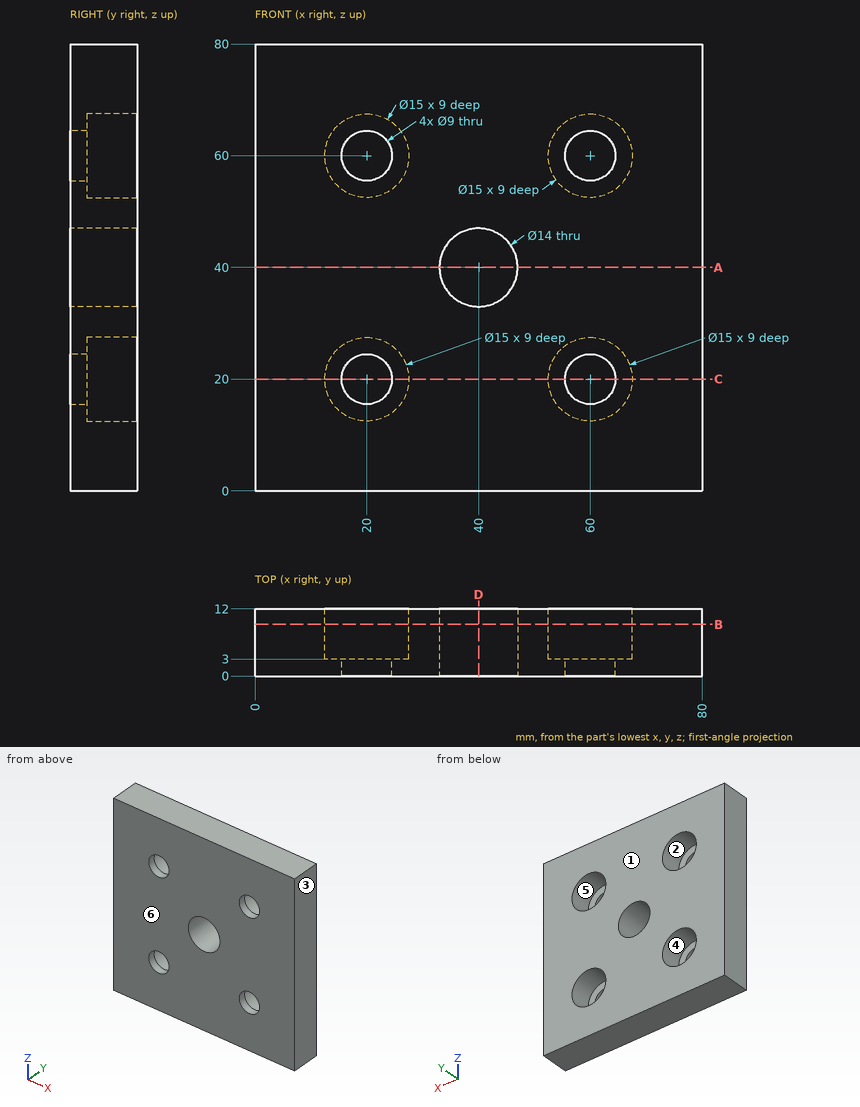
Geometry check sheet. Reference: drawing and pictorial views, mm from the part's lowest x, y, z. A direction names the side the tool comes from. Give positions to 0.01 mm unless a question says otherwise; leave off trailing zeros. Write each loop counter-clockwise with the first axis right and the second up, starting at its lowest first coordinate (ties: lowest second). Pieces come first, ordered by that corner, then holes. Notation, with made-up numbers: M -16,0.5 L -10,0.5 A26 cw -10,16.5 Z; hole C 4,-30 d2. An arc over 180 degrees is marked long. Put each result on its own line as item: value. Start each with the question number.
1. Scan lines: line 1 along X through (y, z) = (2.05, 20); line 2 along X through (y, z) = (7.75, 20); line 3 along Z through (x, y) = (39.5, 7.75). Record each from-to range of solid material in increasing order. Write a range as [from, to].
2. Section check A-A (z = 40). Record the cut outline in (x, y).
3. Go/stop test with flat-tipped pins: pin 1 Ø12.5 at (x, z) = (40, 40) entering from +Y; pin 2 Ø12 at (x, z) = (17.5, 16.5) entering from +Y; pin 3 Ø4.5 at (x, z) = (16.5, 63) entering from +Y. Record where each tip stops, or that it passes through.
4. Section check C-C (z = 20). Record the cut outline in (x, y), and give its area (3 significant figures).
5. Set-up check for the marked faces 1 and 2: record each of +Z, -Z, +X, -X, +Y, -Y from which the full face is reachable in a straight line by a thin tool's end or side.
6. Draft check along X on the marked faces 3, 4, 5 and 6. Enter one of: +X half, -X half, draft (parallel to the pull), parting line (faces both ways), or undercut.
7. Section check D-D (x = 40). Record the cut outline in (y, z), and give its area (3 significant figures).
8. Section check B-B (y = 9.25). Record the cut outline in (x, z), and give its area (3 significant figures).
Answer list:
1. line 1: [0, 15.5], [24.5, 55.5], [64.5, 80]
1. line 2: [0, 12.5], [27.5, 52.5], [67.5, 80]
1. line 3: [0, 33.02], [46.98, 80]
2. outline: M 0,0 L 33,0 L 33,12 L 0,12 Z; M 47,0 L 80,0 L 80,12 L 47,12 Z
3. pin 1: through
3. pin 2: y = 12
3. pin 3: y = 3
4. outline: M 0,0 L 15.5,0 L 15.5,3 L 12.5,3 L 12.5,12 L 0,12 Z; M 24.5,0 L 55.5,0 L 55.5,3 L 52.5,3 L 52.5,12 L 27.5,12 L 27.5,3 L 24.5,3 Z; M 64.5,0 L 80,0 L 80,12 L 67.5,12 L 67.5,3 L 64.5,3 Z
4. area: 636 mm2
5. face 1: +Z, -Z, +X, -X, +Y
5. face 2: +Y
6. face 3: +X half
6. face 4: undercut
6. face 5: undercut
6. face 6: draft
7. outline: M 0,0 L 12,0 L 12,33 L 0,33 Z; M 0,47 L 12,47 L 12,80 L 0,80 Z
7. area: 792 mm2
8. outline: M 0,0 L 80,0 L 80,80 L 0,80 Z; hole C 20,20 d15; hole C 20,60 d15; hole C 40,40 d14; hole C 60,20 d15; hole C 60,60 d15
8. area: 5,540 mm2
